```python
from build123d import *

# Parameters (mm, degrees)
F0_W      = 25.4
F0_H      = 50.8
F1_DEPTH  = 152.4
F2_R      = 12.7
F4_DEPTH  = 152.401
F5_W      = 76.2
F5_H      = 12.7
F6_DEPTH  = 127.001
F7_R      = 6.35
F8_DEPTH  = 50.801
F9_R      = 38.1
F10_DEPTH = 25.401


with BuildPart() as f1:
    # F0 (on Right) → F1 (new body)
    with BuildSketch(Plane.YZ):
        Polygon((-111.00142, 50.8), (-111.00142, 0), (15.99858, 0), (15.99858, 50.8), (-9.40142, 50.8), align=None)
        with Locations((3.29858, 76.2)):
            Rectangle(F0_W, F0_H)
    extrude(amount=F1_DEPTH)

    # F2
    f2_edges = [f1.edges().sort_by_distance(p)[0] for p in [
        (152.4, 3.29858, 101.6),
        (0, 3.29858, 101.6),
    ]]
    fillet(f2_edges, radius=F2_R)

    # F3 (on face) → F4 (cut, through all)
    with BuildSketch(Plane.YZ.offset(152.4)):
        Polygon((-37.97642, 50.8), (-57.02642, 50.8), (-57.02642, 38.1), (-72.90142, 38.1), (-72.90142, 25.4), (-22.10142, 25.4), (-22.10142, 38.1), (-37.97642, 38.1), align=None)
    extrude(amount=-F4_DEPTH, mode=Mode.SUBTRACT)

    # F5 (on face) → F6 (cut, through all)
    with BuildSketch(Plane.XZ.offset(111.00142)):
        with Locations((76.2, 6.35)):
            Rectangle(F5_W, F5_H)
    extrude(amount=-F6_DEPTH, mode=Mode.SUBTRACT)

    # F7 (on face) → F8 (cut, through all)
    with BuildSketch(Plane.XY.offset(50.8)):
        with Locations((19.05, -91.95142)):
            Circle(F7_R)
        with Locations((133.35, -91.95142)):
            Circle(F7_R)
    extrude(amount=-F8_DEPTH, mode=Mode.SUBTRACT)

    # F9 (on face) → F10 (cut, through all)
    with BuildSketch(Plane.XZ.offset(9.40142)):
        with Locations((76.2, 101.6)):
            Circle(F9_R)
    extrude(amount=-F10_DEPTH, mode=Mode.SUBTRACT)


solid = f1.part
```
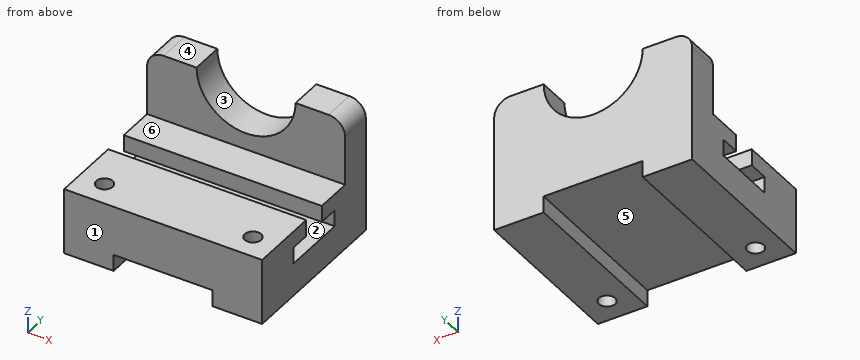
For this review, take the finished solid that the model builds, in its own axes (mm). Face numbers are marked on the shaded views. A direction names the side the tool comes from. Round coordinates to 2 decimals unless told otherwise and drop trailing zeros. Write each loop counter-clockwise with the first axis right and the second up, starting at its lowest first coordinate (ties: lowest second). Pieces come first, ordered by that corner, then holes. Notation, with made-up numbers: M 88,-6.5 L 115,-6.5 A32 ccw 115,27.5 Z; hole C 37.25,4 d5. An arc over 180 degrees is marked long. One line per item, written item: value. Start each with the question number.
(1) The part is to be moulded in two halves that separate along Y. For the marked faces 1, 2 and 3, say which applies: released by +Y, released by -Y, zero draft, split by the parting line, or undercut.
(2) We need section A-A (y = -67.5). Give the boundary of the cut face in (x, z), and give its area (3 significant figures).
(3) We need section D-D (z = 77). Give the boundary of the cut face in (x, y).
(4) Wall thickness on line 1 (Y direction, x = 19.05, z = 13.5); line 2 (Y direction, x = 133, z = 33); line 3 (Z direction, x = 114.5, y = -57.5): over which ranges is each line inside the solid? List them lowest first.
(5) Insertion check: pin 1 (23 mm diameter, centred on x = 84.5, y = -64, fed in from -Z); pin 2 (20.5 mm diameter, centred on x = 133.35, y = -91.95, fed in from -Z); pin 3 (16.5 mm diameter, centred on x = 19.05, y = -91.95, fed in from +Z); pin 4 (6 mm diameter, centred on x = 22.5, z = 73, fed in from -Y). Each pin has a flat end and moves straight along its axis. Give the tip position at first contact, or say it passes through.
(6) We need section C-C (x = 76.2). Give the boundary of the cut face in (y, z).
(7) Machinability: for the marked faces 4, 5 and 6, which of the approach directions +Z, -Z, +X, -X, +Y, -Y give a long, thin tool a straight path to every point of the face, cutting with its end or side? Answer none if there is none.
(8) We need section B-B (x = 19.05). Give the boundary of the cut face in (y, z).
Result:
1. face 1: released by -Y
1. face 2: undercut
1. face 3: zero draft
2. outline: M 0,0 L 38.1,0 L 38.1,12.7 L 114.3,12.7 L 114.3,0 L 152.4,0 L 152.4,25.4 L 0,25.4 Z; M 0,38.1 L 152.4,38.1 L 152.4,50.8 L 0,50.8 Z
2. area: 4,840 mm²
3. outline: M 0,-9.4 L 47.11,-9.4 L 47.11,16 L 0,16 Z; M 105.29,-9.4 L 152.4,-9.4 L 152.4,16 L 105.29,16 Z
4. line 1: -111 to -98.3, -85.6 to 16
4. line 2: -111 to -98.29, -85.61 to -72.9, -22.1 to 16
4. line 3: 0 to 25.4, 38.1 to 50.8
5. pin 1: z = 12.7
5. pin 2: z = 0
5. pin 3: z = 50.8
5. pin 4: y = -9.4
6. outline: M -111,12.7 L 16,12.7 L 16,63.5 L -9.4,63.5 L -9.4,50.8 L -37.98,50.8 L -37.98,38.1 L -22.1,38.1 L -22.1,25.4 L -72.9,25.4 L -72.9,38.1 L -57.03,38.1 L -57.03,50.8 L -111,50.8 Z
7. face 4: +Z, +X, -X, +Y, -Y
7. face 5: -Z, +Y, -Y
7. face 6: +Z, +X, -X, -Y
8. outline: M -111,0 L -98.3,0 L -98.3,50.8 L -111,50.8 Z; M -85.6,0 L 16,0 L 16,101.6 L -9.4,101.6 L -9.4,50.8 L -37.98,50.8 L -37.98,38.1 L -22.1,38.1 L -22.1,25.4 L -72.9,25.4 L -72.9,38.1 L -57.03,38.1 L -57.03,50.8 L -85.6,50.8 Z
